Check sheet for the modelled part. Datum: model origin and axes. Units: mm. Round coordinates to 2 decimals unless told otherwise and drop trailing zeros. Loops run counter-clockwise (first coordinate to the right, second up) from the corner with the lowest first, then second, coordinate; pieces in that order, holes last. Notation, with made-up numbers: (36, 10) - (68, 10) arc R27 ccw to (68, 29) - close; hole circle Ø6 at (18, -37.5). An arc over 180 degrees is marked (long way). Put each result on its own line as item: value. Start each with the question number.
Item 1: Section check A-A, the plane y = 50. Record the cut outline in (x, z).
Item 2: Section check B-B, the plane x = 5. Record the cut outline in (y, z), and give its area (3 significant figures).
Item 3: Gauge pin test, flat ends, axial feed: pin 1 Ø3 at (x, y) = (29.5, 10) entering from -Z; pin 2 Ø3 at (x, y) = (5, 50) entering from +Z. Record the tip position at first contact, or that the pin passes through.
Item 4: Draft check along X on faces 1 (the cylindrical face through (66.6, 49.6, 1.5)), 2 (the flat face through (35, 28, 3)), 3 (the cylindrical face through (69.14, 54.1, 1.52)). Enter one of: pulls with the +X half, pulls with the -X half, needs draft (parallel to the pull), parting line crosses it, or undercut.
Item 5: Material ranges on line 1 along Y through (x, z) = (65, 1.25); line 2 along X through (y, z) = (5, 1.85); line 3 along X through (y, z) = (49, 1.8), recorded low to high.
Autodesk Inventor part; units mm, degrees
ref_plane "YZ Plane" through (0, 0, 0) normal (1, 0, 0) x (0, 1, 0)
ref_plane "XZ Plane" through (0, 0, 0) normal (0, 1, 0) x (-1, 0, 0)
ref_plane "XY Plane" through (0, 0, 0) normal (0, 0, 1) x (1, 0, 0)
sketch "Sketch1" plane through (0, 0, 0) normal (0, 0, 1) x (1, 0, 0)
  line L0 (0, 0) -> (70, 0)
  line L1 (70, 0) -> (70, 55)
  line L2 (70, 55) -> (0, 55)
  line L3 (0, 55) -> (0, 0)
  point P0 (5, 50)
  point P1 (65, 50)
  point P2 (65, 5)
  point P3 (5, 5)
  dimension "d0" = 70
  dimension "d1" = 55
  dimension "d13" = 5
  dimension "d14" = 5
  dimension "d18" = 60
  dimension "d19" = 45
extrude "Extrusion1" add sketch "Sketch1" along normal blind 3
sketch "Sketch3" plane through (0, 0, 0) normal (0, 0, 1) x (1, 0, 0)
  line L0 (0, 0) -> (70, 0)
  line L1 (70, 0) -> (70, 55)
  line L2 (70, 55) -> (0, 55)
  line L3 (0, 55) -> (0, 0)
  point P0 (5, 50)
  point P1 (65, 50)
  point P2 (65, 5)
  point P3 (5, 5)
  dimension "d20" = 70
  dimension "d21" = 55
  dimension "d22" = 5
  dimension "d23" = 5
  dimension "d24" = 60
  dimension "d25" = 45
hole "Hole1" at (5, 50, 0) at (65, 50, 0) at (65, 5, 0) at (5, 5, 0) direction (0, 0, 1) diameter 3.3 end through all
fillet "Fillet1" radius 3 4 edges at (70, 55, 1.5) (70, 0, 1.5) (0, 0, 1.5) (0, 55, 1.5)
sketch "Sketch4" plane through (0, 0, 3) normal (0, 0, 1) x (1, 0, 0)
  arc A0 (3, 55) -> (0, 52) centre (3, 52) ccw
  line L0 (0, 52) -> (0, 3)
  arc A1 (0, 3) -> (3, 0) centre (3, 3) ccw
  line L1 (3, 0) -> (67, 0)
  arc A2 (67, 0) -> (70, 3) centre (67, 3) ccw
  line L2 (70, 3) -> (70, 52)
  arc A3 (70, 52) -> (67, 55) centre (67, 52) ccw
  line L3 (67, 55) -> (3, 55)
  circle A4 centre (65, 5) radius 1.65
  circle A5 centre (5, 50) radius 1.65
  circle A6 centre (65, 50) radius 1.65
  circle A7 centre (5, 5) radius 1.65
  point P0 (0, 0)
properties part number "BasePixhawk"
Check result:
1. outline: (0, 0) - (3.35, 0) - (3.35, 3) - (0, 3) - close; (6.65, 0) - (63.35, 0) - (63.35, 3) - (6.65, 3) - close; (66.65, 0) - (70, 0) - (70, 3) - (66.65, 3) - close
2. outline: (0, 0) - (3.35, 0) - (3.35, 3) - (0, 3) - close; (6.65, 0) - (48.35, 0) - (48.35, 3) - (6.65, 3) - close; (51.65, 0) - (55, 0) - (55, 3) - (51.65, 3) - close
2. area: 145 mm²
3. pin 1: z = 0
3. pin 2: through
4. face 1: undercut
4. face 2: needs draft
4. face 3: pulls with the +X half
5. line 1: 0 to 3.35, 6.65 to 48.35, 51.65 to 55
5. line 2: 0 to 3.35, 6.65 to 63.35, 66.65 to 70
5. line 3: 0 to 3.69, 6.31 to 63.69, 66.31 to 70
